Job drawing, mm, ordinate dimensions from the low corner. One solid piece. A direction names the side the tool comes from. Give positions to 0.01 mm unless a question says otherwise; leave off trailing zeros. Write each loop counter-clockwise with the first axis right and the second up, starting at its lowest first coordinate (ties: lowest second). Pieces come first, ordered by that corner, then holes. Notation, with made-up numbers: (55, 46) - (59, 46) arc R20 ccw to (59, 71) - close; hole circle Ø2 at (77, 11). An arc over 180 degrees is marked (long way). Answer in a Markdown table with one row per item. Add a question column.
1. Probe line 1 along Y through (x, z) = (464, 27) (1 decimal); line 2 along X through (y, z) = (70, 27); line 3 along X through (y, z) = (136.5, 25). List the from-to ranges inside material, lowest first.
2. Band-saw the part on B-B on y = 44. Write the cut outline in (x, z), plus the area to 3 significant figures.
3. Drop flat-ended pins along their axis: pin 1 Ø7 at (x, z) = (272.5, 29.5) entering from +Y; pin 2 Ø12.5 at (x, z) = (65.5, 13) entering from -Y; pin 3 Ø7 at (x, z) = (388, 29.5) entering from -Y (1 decimal). Give the stop position or say it passes through.
4. Band-saw the part on C-C on z = 21. Write the cut outline in (x, y).
5. Pull direction X, two halves, no side cores. Call the marked faces 3, 4 and 5: released by +X, released by -X, zero draft, split by the parting line, or undercut.
6. Band-saw the part on D-D on x = 131. Write the cut outline in (y, z), plus the area to 3 significant figures.
7. Which spindle directions (+Z, -Z, +X, -X, +Y, -Y) get a long thin tool onto all of the face, cutting with end or side? Do the marked faces 1 and 2. Say none if no direction does.
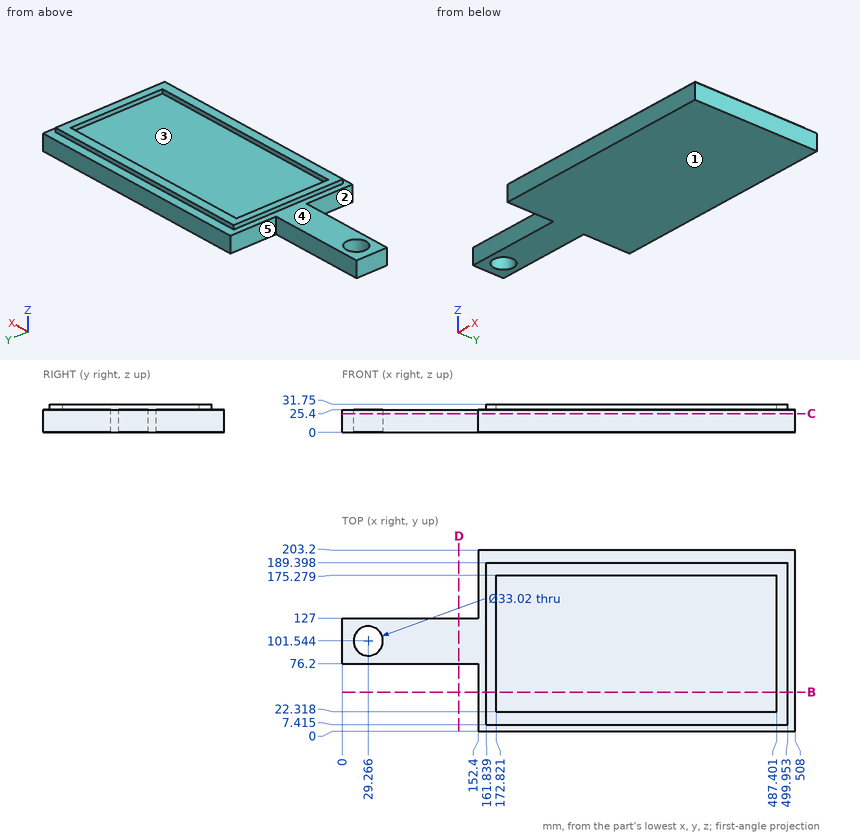
Values:
| question | item | result |
|---|---|---|
| 1 | line 1 | y = 7.4 to 22.3, 175.3 to 189.4 |
| 1 | line 2 | x = 161.84 to 172.82, 487.4 to 499.95 |
| 1 | line 3 | x = 152.4 to 508 |
| 2 | outline | (152.4, 0) - (508, 0) - (508, 25.4) - (499.95, 25.4) - (499.95, 31.75) - (487.4, 31.75) - (487.4, 25.4) - (172.82, 25.4) - (172.82, 31.75) - (161.84, 31.75) - (161.84, 25.4) - (152.4, 25.4) - close |
| 2 | area | 9,180 mm² |
| 3 | pin 1 | stops at y = 189.4 |
| 3 | pin 2 | stops at y = 76.2 |
| 3 | pin 3 | stops at y = 7.4 |
| 4 | outline | (0, 76.2) - (152.4, 76.2) - (152.4, 0) - (508, 0) - (508, 203.2) - (152.4, 203.2) - (152.4, 127) - (0, 127) - close; hole circle Ø33.02 at (29.27, 101.54) |
| 5 | face 3 | undercut |
| 5 | face 4 | zero draft |
| 5 | face 5 | released by -X |
| 6 | outline | (76.2, 0) - (127, 0) - (127, 25.4) - (76.2, 25.4) - close |
| 6 | area | 1,290 mm² |
| 7 | face 1 | -Z, +X, -X, +Y, -Y |
| 7 | face 2 | +Z, -Z, -X, -Y |
